from build123d import *

# Parameters (mm, degrees)
MODEL_R             = 3.55
MODEL_R_2           = 1.5
BOSS_EXTRUDE1_DEPTH = 2.55


with BuildPart() as part:
    # Model → Boss-Extrude1 (new body)
    with BuildSketch(Plane.XY):
        with BuildLine():
            Line((-4, 121), (-4, 7.745966692))
            ThreePointArc((-4, 7.745966692), (-4.317541634, 5.245966692), (-5.25, 2.90473751))
            ThreePointArc((-5.25, 2.90473751), (-6, 0), (-5.25, -2.90473751))
            ThreePointArc((-5.25, -2.90473751), (-4.317541634, -5.245966692), (-4, -7.745966692))
            Line((-4, -7.745966692), (-4, -13.8))
            ThreePointArc((-4, -13.8), (0, -17.8), (4, -13.8))
            Line((4, -13.8), (4, -7.745966692))
            ThreePointArc((4, -7.745966692), (4.317541634, -5.245966692), (5.25, -2.90473751))
            ThreePointArc((5.25, -2.90473751), (6, 0), (5.25, 2.90473751))
            ThreePointArc((5.25, 2.90473751), (4.317541634, 5.245966692), (4, 7.745966692))
            Line((4, 7.745966692), (4, 121))
            ThreePointArc((4, 121), (0, 125), (-4, 121))
        make_face()
        Circle(MODEL_R, mode=Mode.SUBTRACT)
        with Locations((0, 121)):
            Circle(MODEL_R_2, mode=Mode.SUBTRACT)
        with BuildLine():
            Line((-1, -10.1), (-1, -13.8))
            ThreePointArc((-1, -13.8), (0, -14.8), (1, -13.8))
            Line((1, -13.8), (1, -10.1))
            ThreePointArc((1, -10.1), (0, -9.1), (-1, -10.1))
        make_face(mode=Mode.SUBTRACT)
        with BuildLine():
            Line((-1, 15.1), (-1, 10.1))
            ThreePointArc((-1, 10.1), (0, 9.1), (1, 10.1))
            Line((1, 10.1), (1, 15.1))
            ThreePointArc((1, 15.1), (0, 16.1), (-1, 15.1))
        make_face(mode=Mode.SUBTRACT)
    extrude(amount=BOSS_EXTRUDE1_DEPTH)


solid = part.part
The model under review builds one solid part; all positions refer to its coordinate system, in mm. A direction names the side the tool comes from. Give positions to 0.01 mm unless a question says otherwise; leave off trailing zeros. Loops run counter-clockwise (first coordinate to the right, second up) from the corner with the lowest first, then second, coordinate; pieces in that order, holes last. Notation, with made-up numbers: (-29.75, -5.75) -> (14.25, -5.75) arc R19 cw to (14.25, -1.75) -> close; hole circle Ø3 at (71.5, -6.5). An arc over 180 degrees is marked (long way). Put each result on its own line as item: value. Start each with the question number.
1. For faces 4 (the face through (-4, 65, 1)), 5 (the face through (4, -11, 1)), 6 (the face through (4, 64, 1)), 7 (the face through (-1, -12, 1)), list the 3-axis set-ups (+Z, -Z, +X, -X, +Y, -Y) from which the entire face can be reached by the end or side of a thin tool; tool diameter is ignored.
2. We need section B-B on z = 1.4. State the section outline as (x, y) points, then the cut area to 3 significant figures.
3. We need section C-C on y = 59.5. State the section outline as (x, z) points.
4. Wall thickness on probe 1 along Y at (x, z) = (0, 0.8); probe 2 along X at (y, z) = (121, 1.35); probe 3 along X at (y, z) = (74, 2.1): over which ranges is each line inside the solid? List them lowest first.
5. Mouldability with a two-part tool opening along Y and no side actions: class faces 1 (the face through (1, -12, 1)), 2 (the face through (-4, -11, 1)), 3 (the face through (-0.1, -17.8, 1.3)) as released by +Y, released by -Y, zero draft, split by the parting line, or undercut.
6. Clearance check with flat-ended pins moving along their axes: P1, Ø1.3, axis at y = -10, z = 1.5, coming from the -X side; P2, Ø1.3, axis at y = -12.5, z = 1.5, coming from the +X side; P3, Ø1, axis at y = 6.5, z = 0.5, coming from the -X side. State where each tip first meets the part, or that it passes through.
7. We need section A-A on y = 0. State the section outline as (x, z) points, then the cut area to 3 significant figures.
Determined:
1. face 4: +Z, -Z, -X, +Y
1. face 5: +Z, -Z, +X, -Y
1. face 6: +Z, -Z, +X, +Y
1. face 7: +Z, -Z
2. outline: (-5.25, -2.9) arc R10 cw to (-4, -7.75) -> (-4, -13.8) arc R4 ccw to (4, -13.8) -> (4, -7.75) arc R10 cw to (5.25, -2.9) arc R6 ccw to (5.25, 2.9) arc R10 cw to (4, 7.75) -> (4, 121) arc R4 ccw to (-4, 121) -> (-4, 7.75) arc R10 cw to (-5.25, 2.9) arc R6 ccw to start; hole circle Ø7.1 at (0, 0); hole circle Ø3 at (0, 121); hole (-1, -13.8) arc R1 ccw to (1, -13.8) -> (1, -10.1) arc R1 ccw to (-1, -10.1) -> close; hole (-1, 10.1) arc R1 ccw to (1, 10.1) -> (1, 15.1) arc R1 ccw to (-1, 15.1) -> close
2. area: 1,090 mm^2
3. outline: (-4, 0) -> (4, 0) -> (4, 2.55) -> (-4, 2.55) -> close
4. probe 1: -17.8 to -14.8, -9.1 to -3.55, 3.55 to 9.1, 16.1 to 119.5, 122.5 to 125
4. probe 2: -4 to -1.5, 1.5 to 4
4. probe 3: -4 to 4
5. face 1: undercut
5. face 2: zero draft
5. face 3: released by -Y
6. P1: x = -4
6. P2: x = 4
6. P3: x = -4.15
7. outline: (-6, 0) -> (-3.55, 0) -> (-3.55, 2.55) -> (-6, 2.55) -> close; (3.55, 0) -> (6, 0) -> (6, 2.55) -> (3.55, 2.55) -> close
7. area: 12.5 mm^2
